Source: CAD feature listing. Evaluate the final solid. Frame: model axes, mm. A direction names the side the tool comes from. Round coordinates to 2 decimals unless told otherwise and drop trailing zeros. Order: outer loops, then holes, each group sorted by start corner. A loop starts at its lowest first (then second) coordinate and runs counter-clockwise, first axis right, second up. Notation, with made-up numbers: (85.25, 50.25) -> (132.25, 50.25) arc R21 ccw to (132.25, 56.25) -> close; hole circle Ø5 at (29.25, 46). An arc over 180 degrees is marked (long way). Answer as CSV lines item,"result".
from build123d import *

# Parameters (mm, degrees)
SKETCH1_W                  = 5
SKETCH1_H                  = 26
EXTRUDE1_DEPTH             = 7
F_2_7_2_7_DIAMETER_HOLE1_D = 2.7
EXTRUDE3_REACH             = 17.588
SKETCH8_W                  = 5
SKETCH8_H                  = 5
FILLET1_R                  = 1
FILLET2_R                  = 1
EXTRUDE4_REACH             = 17.588


with BuildPart() as part:
    # Sketch1 → Extrude1 (new body)
    with BuildSketch(Plane.XY):
        Rectangle(SKETCH1_W, SKETCH1_H)
    extrude(amount=EXTRUDE1_DEPTH)

    # Ø2.7 (2.7) Diameter Hole1 (through all)
    with Locations(Plane(origin=(0, 0, 0), x_dir=(-1, 0, 0), z_dir=(0, 0, -1))):
        with Locations((0, 10.5), (0, -10.5)):
            Hole(F_2_7_2_7_DIAMETER_HOLE1_D / 2)

    # Extrude3: up to this face of the body (flat: up to its plane)
    extrude3_end = Plane(part.part.faces().sort_by_distance((-2.5, 0, 3.5))[0])
    # Sketch8 → Extrude3 (cut, up to the picked face)
    with BuildSketch(Plane(origin=(2.5, 0, 0), x_dir=(0, 0, -1), z_dir=(1, 0, 0)), mode=Mode.PRIVATE) as extrude3_sk1:
        with Locations((-4.5, -10.5)):
            Rectangle(SKETCH8_W, SKETCH8_H)
    extrude3_tool1 = split(extrude(extrude3_sk1.sketch, amount=-EXTRUDE3_REACH, mode=Mode.PRIVATE), bisect_by=extrude3_end, keep=Keep.BOTH, mode=Mode.PRIVATE)
    # Sketch8 → Extrude3 (cut, up to the picked face)
    with BuildSketch(Plane(origin=(2.5, 0, 0), x_dir=(0, 0, -1), z_dir=(1, 0, 0)), mode=Mode.PRIVATE) as extrude3_sk2:
        with Locations((-4.5, 10.5)):
            Rectangle(SKETCH8_W, SKETCH8_H)
    extrude3_tool2 = split(extrude(extrude3_sk2.sketch, amount=-EXTRUDE3_REACH, mode=Mode.PRIVATE), bisect_by=extrude3_end, keep=Keep.BOTH, mode=Mode.PRIVATE)
    add(extrude3_tool1.solids().sort_by(Axis((2.5, -10.5, 4.5), (-1, 0, 0)))[0], mode=Mode.SUBTRACT)
    add(extrude3_tool2.solids().sort_by(Axis((2.5, 10.5, 4.5), (-1, 0, 0)))[0], mode=Mode.SUBTRACT)

    # Fillet1
    fillet1_edges = [part.edges().sort_by_distance(p)[0] for p in [
        (2.5, 0, 7),
        (-2.5, 0, 7),
    ]]
    fillet(fillet1_edges, radius=FILLET1_R)

    # Fillet2
    fillet2_edges = [part.edges().sort_by_distance(p)[0] for p in [
        (2.5, -13, 1),
        (-2.5, -13, 1),
        (-2.5, 13, 1),
        (2.5, 13, 1),
    ]]
    fillet(fillet2_edges, radius=FILLET2_R)

    # Extrude4: up to this face of the body (flat: up to its plane)
    extrude4_end = Plane(part.part.faces().sort_by_distance((2.5, 0, 2.714285714))[0])
    # Sketch9 → Extrude4 (cut, up to the picked face)
    with BuildSketch(Plane.ZY.offset(2.5), mode=Mode.PRIVATE) as extrude4_sk1:
        with BuildLine():
            Line((2, 8), (3.710100717, 7.377574242))
            ThreePointArc((3.710100717, 7.377574242), (6.095760221, 5.546993319), (7, 2.679111138))
            Line((7, 2.679111138), (7, 8))
            Line((7, 8), (2, 8))
        make_face()
    extrude4_tool1 = split(extrude(extrude4_sk1.sketch, amount=-EXTRUDE4_REACH, mode=Mode.PRIVATE), bisect_by=extrude4_end, keep=Keep.BOTH, mode=Mode.PRIVATE)
    add(extrude4_tool1.solids().sort_by(Axis((-2.5, 6.831886, 5.650764), (1, 0, 0)))[0], mode=Mode.SUBTRACT)


solid = part.part
1. Section query D-D on y = 4.25. Return loops of the section in (x, z), and give its area (3 significant figures).
Results below:
outline,"(-2.5, 0) -> (2.5, 0) -> (2.5, 6) arc R1 ccw to (2.17, 6.75) -> (-2.17, 6.75) arc R1 ccw to (-2.5, 6) -> close"
area,"33.6 mm2"
2. Reachability of faces 4 (the flat face through (-1, 9, 2)), 5 (the flat face through (0, -8, 5)), 6 (the flat face through (-2.5, 0, 2)) from +Z, -Z, +X, -X, +Y, -Y: full face, straight path, thin tool, end or side. Return the list, or none.
Results below:
face 4,"+Z, +X, -X, +Y"
face 5,"+Z, +X, -X, -Y"
face 6,"+Z, -Z, -X, +Y, -Y"
3. Line query: L1, parallel to Y at x = 0, z = 0.8; L2, parallel to Z at x = 1.5, y = 10.5; L3, parallel to Z at x = 0.65, y = 4.5. Output: solid intervals per line, ascending. Write a range as [from, to].
Results below:
L1,"[-13, -11.85], [-9.15, 9.15], [11.85, 13]"
L2,"[0, 2]"
L3,"[0, 6.66]"
4. Mould query, pull axis Y, two halves, no side actions, for faces 1 (the cylindrical face through (2.199, -1.065, 6.715)), 2 (the flat face through (0, 13, 1)), 3 (the cylindrical face through (-0.176, 11.839, 1.014)). Classes: released by +Y, released by -Y, zero draft, split by the parting line, or undercut.
Results below:
face 1,"zero draft"
face 2,"released by +Y"
face 3,"undercut"
5. Section query A-A on x = 0. Return loops of the section in (y, z).
Results below:
outline,"(-13, 0) -> (-11.85, 0) -> (-11.85, 2) -> (-13, 2) -> close; (-9.15, 0) -> (9.15, 0) -> (9.15, 2) -> (8, 2) -> (7.38, 3.71) arc R5 ccw to (2.68, 7) -> (-8, 7) -> (-8, 2) -> (-9.15, 2) -> close; (11.85, 0) -> (13, 0) -> (13, 2) -> (11.85, 2) -> close"
6. Section query B-B on y = 10.5. Return loops of the section in (x, z).
Results below:
outline,"(-2.5, 0) -> (-1.35, 0) -> (-1.35, 2) -> (-2.5, 2) -> close; (1.35, 0) -> (2.5, 0) -> (2.5, 2) -> (1.35, 2) -> close"
7. Pin query (flat end, axial travel): pin 1 (1.5 mm diameter, centred on x = 1, z = 4, fed in from -Y); pin 2 (1.5 mm diameter, centred on x = -1, y = -11, fed in from +Z); pin 3 (3 mm diameter, centred on x = 1.5, z = 5.5, fed in from +Y). Return the tip coordinate at first contact, or that it passes through.
Results below:
pin 1,"y = -8"
pin 2,"z = 2"
pin 3,"y = 7.26"
8. Section query C-C on z = 5.25. Return loops of the section in (x, y).
Results below:
outline,"(-2.5, -8) -> (2.5, -8) -> (2.5, 6.48) -> (-2.5, 6.48) -> close"
